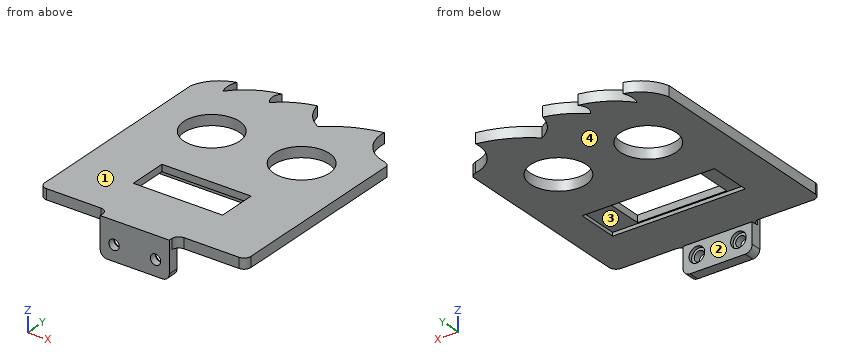
```python
from build123d import *

# Parameters (mm, degrees)
MODEL_R                 = 8.05
MODEL_W                 = 25.8
MODEL_H                 = 11.3
SALIENTE_EXTRUIR1_DEPTH = 3
CROQUIS2_W              = 20
CROQUIS2_H              = 3
SALIENTE_EXTRUIR2_DEPTH = 8
CROQUIS3_R              = 1.5
CORTAR_EXTRUIR1_DEPTH   = 3
CROQUIS4_R              = 2.25
CORTAR_EXTRUIR2_DEPTH   = 1
REDONDEO1_R             = 2
CROQUIS5_W              = 38.3
CROQUIS5_H              = 12.1
CORTAR_EXTRUIR3_DEPTH   = 1


with BuildPart() as part:
    # Model → Saliente-Extruir1 (new body)
    with BuildSketch(Plane.XY):
        with BuildLine():
            Line((50.589823504, -56.020997464), (70.589823504, -56.020997464))
            Line((70.589823504, -56.020997464), (70.589823504, -55.020997464))
            ThreePointArc((70.589823504, -55.020997464), (71.175609941, -53.606783901), (72.589823504, -53.020997464))
            Line((72.589823504, -53.020997464), (88.542347513, -53.020997464))
            ThreePointArc((88.542347513, -53.020997464), (89.956561076, -52.435211026), (90.542347513, -51.020997464))
            Line((90.542347513, -51.020997464), (90.542347513, 2.706709465))
            ThreePointArc((90.542347513, 2.706709465), (89.85153081, 3.480899542), (88.938302171, 3.973455574))
            ThreePointArc((88.938302171, 3.973455574), (82.554576883, 7.967186508), (80.590162534, 15.236499516))
            ThreePointArc((80.590162534, 15.236499516), (73.013912202, 12.831206377), (66.42202871, 8.389126209))
            ThreePointArc((66.42202871, 8.389126209), (62.462620999, 11.66270114), (60.385206297, 16.361376528))
            ThreePointArc((60.385206297, 16.361376528), (55.037159481, 14.426569266), (50.459652092, 11.051438157))
            ThreePointArc((50.459652092, 11.051438157), (49.412602259, 13.546636971), (50.436598222, 16.051385009))
            ThreePointArc((50.436598222, 16.051385009), (43.797798117, 13.634815248), (38.469001196, 8.99613013))
            ThreePointArc((38.469001196, 8.99613013), (37.974300587, 11.673196605), (38.616025483, 14.318872844))
            ThreePointArc((38.616025483, 14.318872844), (33.704473328, 11.607826814), (30.85334667, 6.776244059))
            Line((30.85334667, 6.776244059), (30.85334667, -51.020997464))
            ThreePointArc((30.85334667, -51.020997464), (31.439133108, -52.435211026), (32.85334667, -53.020997464))
            Line((32.85334667, -53.020997464), (48.589823504, -53.020997464))
            ThreePointArc((48.589823504, -53.020997464), (50.004037066, -53.606783901), (50.589823504, -55.020997464))
            Line((50.589823504, -55.020997464), (50.589823504, -56.020997464))
        make_face()
        with Locations((47.698959583, -8.020997464)):
            Circle(MODEL_R, mode=Mode.SUBTRACT)
        with Locations((73.698959582, -8.020997464)):
            Circle(MODEL_R, mode=Mode.SUBTRACT)
        with Locations((60.589823504, -33.326919867)):
            Rectangle(MODEL_W, MODEL_H, mode=Mode.SUBTRACT)
    extrude(amount=SALIENTE_EXTRUIR1_DEPTH)

    # Croquis2 → Saliente-Extruir2 (add)
    with BuildSketch(Plane(origin=(0, 0, 0), x_dir=(-1, 0, 0), z_dir=(0, 0, -1))):
        with Locations((-60.589823504, -54.520997464)):
            Rectangle(CROQUIS2_W, CROQUIS2_H)
    extrude(amount=SALIENTE_EXTRUIR2_DEPTH)

    # Croquis3 → Cortar-Extruir1 (cut)
    with BuildSketch(Plane(origin=(0, -53.020997464, 0), x_dir=(1, 0, 0), z_dir=(0, 1, 0))):
        with Locations((66.589823504, 3.5)):
            Circle(CROQUIS3_R)
        with Locations((54.589823504, 3.5)):
            Circle(CROQUIS3_R)
    extrude(amount=-CORTAR_EXTRUIR1_DEPTH, mode=Mode.SUBTRACT)

    # Croquis4 → Cortar-Extruir2 (cut)
    with BuildSketch(Plane(origin=(0, -53.020997464, 0), x_dir=(1, 0, 0), z_dir=(0, 1, 0))):
        with Locations((66.589823504, 3.5)):
            Circle(CROQUIS4_R)
        with Locations((54.589823504, 3.5)):
            Circle(CROQUIS4_R)
    extrude(amount=-CORTAR_EXTRUIR2_DEPTH, mode=Mode.SUBTRACT)

    # Redondeo1
    redondeo1_edges = [part.edges().sort_by_distance(p)[0] for p in [
        (50.589823504, -54.520997464, -8),
        (70.589823504, -54.520997464, -8),
    ]]
    fillet(redondeo1_edges, radius=REDONDEO1_R)

    # Croquis5 → Cortar-Extruir3 (cut)
    with BuildSketch(Plane(origin=(0, 0, 0), x_dir=(-1, 0, 0), z_dir=(0, 0, -1))):
        with Locations((-61.789823504, -33.326919867)):
            Rectangle(CROQUIS5_W, CROQUIS5_H)
    extrude(amount=-CORTAR_EXTRUIR3_DEPTH, mode=Mode.SUBTRACT)


solid = part.part
```
CAD build for the part. Positions are in the model's coordinates, mm. Face numbers are marked on the shaded views. A direction names the side the tool comes from. Coordinates: 2 decimals unless noted, no trailing zeros. Order: outer loops, then holes, each group sorted by start corner. A loop starts at its lowest first (then second) coordinate and runs counter-clockwise, first axis right, second up. Notation, with made-up numbers: M 37,-3 L 48,-3 A25 cw 48,28 Z; hole C -11.75,0 d10. An arc over 180 degrees is marked long. Write each question's results on one line, items separated by ' | '. Start each with the question number.
Q1. Cut at B-B (y = -29). List the corners of the cut face in (x, z).
Q2. Drill centre lines: probe 1 along Y at (x, z) = (48, 1.25); probe 2 along Z at (x, y) = (87, -10); probe 3 along Y at (x, z) = (53.5, 0.75). Where is each one in solid material? Low to high. Write a range as from..to.
Q3. Which spindle directions (+Z, -Z, +X, -X, +Y, -Y) get a long thin tool onto all of the face, cutting with end or side? Do the marked faces 1 and 2. Say none if no direction does.
Q4. Pull direction X, two halves, no side cores. Call the marked faces 3 and 4: +X half, -X half, draft (parallel to the pull), parting line (faces both ways), or undercut.
Q5. Flat gauge pins, fed straight in: P1, Ø1.5, axis at y = -22, z = -1, coming from the -X side; P2, Ø3.5, axis at x = 55, z = -4, coming from the +Y side; P3, Ø3.5, axis at x = 44, z = 1, coming from the -Y side; P4, Ø3.5, axis at y = -54.5, z = 0.5, coming from the +X side. Where does each tip first touch, or does it go through?
Q6. Cut at A-A (z = -3.5). List the corners of the cut face in (x, y).
Found:
1) outline: M 30.85,0 L 42.64,0 L 42.64,1 L 47.69,1 L 47.69,3 L 30.85,3 Z; M 73.49,1 L 80.94,1 L 80.94,0 L 90.54,0 L 90.54,3 L 73.49,3 Z
2) probe 1: -53.02..-38.98, -27.68..-16.07, 0.02..15.48 | probe 2: 0..3 | probe 3: -56.02..-39.38, -27.28..-13.6, -2.44..13.51
3) face 1: +Z, +X, -X, +Y, -Y | face 2: -Z, +X, -X, +Y
4) face 3: undercut | face 4: draft
5) P1: through | P2: y = -53.02 | P3: y = -53.02 | P4: x = 89.55
6) outline: M 50.59,-56.02 L 53.09,-56.02 L 53.09,-54.02 L 52.34,-54.02 L 52.34,-53.02 L 50.59,-53.02 Z; M 56.09,-56.02 L 65.09,-56.02 L 65.09,-54.02 L 64.34,-54.02 L 64.34,-53.02 L 56.84,-53.02 L 56.84,-54.02 L 56.09,-54.02 Z; M 68.09,-56.02 L 70.59,-56.02 L 70.59,-53.02 L 68.84,-53.02 L 68.84,-54.02 L 68.09,-54.02 Z
